Build history of the part. All positions in model axes, mm. A direction names the side the tool comes from. Round coordinates to 2 decimals unless told otherwise and drop trailing zeros. Order: outer loops, then holes, each group sorted by start corner. A loop starts at its lowest first (then second) coordinate and runs counter-clockwise, first axis right, second up. Notation, with made-up numbers: (38, -14.5) -> (83, -14.5) arc R21 cw to (83, 21.5) -> close; hole circle Ø4 at (89.5, -0.75). An arc over 180 degrees is marked (long way). Answer as a JSON object with one key per item and string values.
from build123d import *

# Parameters (mm, degrees)
SKETCH1_W           = 42
SKETCH1_H           = 42
BOSS_EXTRUDE1_DEPTH = 6
SKETCH2_W           = 39
SKETCH2_H           = 39
CUT_EXTRUDE1_DEPTH  = 3.5
CUT_EXTRUDE2_REACH  = 31.904
SKETCH3_W           = 5
SKETCH3_H           = 7
SKETCH3_W_2         = 13
SKETCH3_H_2         = 6
BOSS_EXTRUDE2_DEPTH = 2
SKETCH5_R           = 1
CUT_EXTRUDE3_DEPTH  = 31.037476592
SKETCH6_R           = 5
BOSS_EXTRUDE3_DEPTH = 8
SKETCH7_R           = 2.5
BOSS_EXTRUDE4_DEPTH = 10
FILLET1_R           = 1


with BuildPart() as part:
    # Sketch1 → Boss-Extrude1 (new body)
    with BuildSketch(Plane(origin=(0, 0, 0), x_dir=(1, 0, 0), z_dir=(0, 1, 0))):
        Rectangle(SKETCH1_W, SKETCH1_H)
    extrude(amount=BOSS_EXTRUDE1_DEPTH)

    # Sketch2 → Cut-Extrude1 (cut)
    with BuildSketch(Plane.XZ):
        Rectangle(SKETCH2_W, SKETCH2_H)
    extrude(amount=-CUT_EXTRUDE1_DEPTH, mode=Mode.SUBTRACT)

    # Sketch3 → Cut-Extrude2 (cut, up to next)
    with BuildSketch(Plane.XZ.offset(-3.5), mode=Mode.PRIVATE) as cut_extrude2_sk1:
        with Locations((-17, 8.5)):
            Rectangle(SKETCH3_W, SKETCH3_H)
    cut_extrude2_tool1 = extrude(cut_extrude2_sk1.sketch, amount=-CUT_EXTRUDE2_REACH, mode=Mode.PRIVATE) & part.part
    # Sketch3 → Cut-Extrude2 (cut, up to next)
    with BuildSketch(Plane.XZ.offset(-3.5), mode=Mode.PRIVATE) as cut_extrude2_sk2:
        with Locations((-6, 16.5)):
            Rectangle(SKETCH3_W_2, SKETCH3_H_2)
    cut_extrude2_tool2 = extrude(cut_extrude2_sk2.sketch, amount=-CUT_EXTRUDE2_REACH, mode=Mode.PRIVATE) & part.part
    add(cut_extrude2_tool1.solids().sort_by_distance((-17, 3.5, 8.5))[0], mode=Mode.SUBTRACT)
    add(cut_extrude2_tool2.solids().sort_by_distance((-6, 3.5, 16.5))[0], mode=Mode.SUBTRACT)

    # Sketch4 → Boss-Extrude2 (add)
    with BuildSketch(Plane.XZ.offset(-3.5)):
        with BuildLine():
            Line((-19.5, 17), (-19.5, 19.5))
            Line((-19.5, 19.5), (-17, 19.5))
            ThreePointArc((-17, 19.5), (-15.232233047, 15.232233047), (-19.5, 17))
        make_face()
        with BuildLine():
            Line((19.5, 19.5), (17, 19.5))
            ThreePointArc((17, 19.5), (15.232233047, 15.232233047), (19.5, 17))
            Line((19.5, 17), (19.5, 19.5))
        make_face()
        with BuildLine():
            Line((-19.5, -19.5), (-17, -19.5))
            ThreePointArc((-17, -19.5), (-15.232233047, -15.232233047), (-19.5, -17))
            Line((-19.5, -17), (-19.5, -19.5))
        make_face()
        with BuildLine():
            Line((19.5, -17), (19.5, -19.5))
            Line((19.5, -19.5), (17, -19.5))
            ThreePointArc((17, -19.5), (15.232233047, -15.232233047), (19.5, -17))
        make_face()
    extrude(amount=BOSS_EXTRUDE2_DEPTH)

    # Sketch5 → Cut-Extrude3 (cut, through all)
    with BuildSketch(Plane.XZ.offset(-1.5)):
        with Locations(Location((-17, 17, 0), (0, 0, 270))):
            Circle(SKETCH5_R)
        with Locations(Location((17, 17, 0), (0, 0, 270))):
            Circle(SKETCH5_R)
        with Locations(Location((17, -17, 0), (0, 0, 270))):
            Circle(SKETCH5_R)
        with Locations(Location((-17, -17, 0), (0, 0, 270))):
            Circle(SKETCH5_R)
    extrude(amount=-CUT_EXTRUDE3_DEPTH, mode=Mode.SUBTRACT)

    # Sketch6 → Boss-Extrude3 (add)
    with BuildSketch(Plane(origin=(0, 6, 0), x_dir=(1, 0, 0), z_dir=(0, 1, 0))):
        with Locations(Location((0, 0, 0), (0, 0, 270))):
            Circle(SKETCH6_R)
    extrude(amount=BOSS_EXTRUDE3_DEPTH)

    # Sketch7 → Boss-Extrude4 (add)
    with BuildSketch(Plane(origin=(0, 14, 0), x_dir=(1, 0, 0), z_dir=(0, 1, 0))):
        with Locations(Location((0, 0, 0), (0, 0, 270))):
            Circle(SKETCH7_R)
    extrude(amount=BOSS_EXTRUDE4_DEPTH)

    # Fillet1
    fillet1_edges = [part.edges().sort_by_distance(p)[0] for p in [
        (0, 6, -5),
        (0, 14, -2.5),
        (0, 24, -2.5),
        (-21, 6, 0),
        (0, 6, 21),
        (-14.5, 4.75, 12),
        (-14.5, 4.75, 5),
        (-19.5, 4.75, 5),
        (-19.5, 4.75, 12),
        (0.5, 4.75, 19.5),
        (0.5, 4.75, 13.5),
        (-12.5, 4.75, 13.5),
        (-12.5, 4.75, 19.5),
        (21, 6, 0),
        (21, 3, 21),
        (-21, 3, 21),
        (-21, 3, -21),
        (21, 3, -21),
        (0, 6, -21),
    ]]
    fillet(fillet1_edges, radius=FILLET1_R)


solid = part.part
1) Probe L1, parallel to X at y = 3.9, z = 17; L2, parallel to X at y = 4.7, z = -17; L3, parallel to X at y = 3, z = 4.5. List the from-to ranges inside material, lowest first. Write a range as from..to.
Checked values:
{"L1": "x = -21..-18, -16..-12.5, 0.5..16, 18..21", "L2": "x = -21..-18, -16..16, 18..21", "L3": "x = -21..-19.5, 19.5..21"}
2) Which spindle directions (+Z, -Z, +X, -X, +Y, -Y) get a long thin tool onto all of the face, cutting with end or side? Do faces 5 (the face through (0, 2, 21)), 6 (the face through (-14.801, 4.768, 11.715)), 7 (the face through (-18, 1.5, 18)). Say none if no direction does.
Checked values:
{"face 5": "+Z, +X, -X, +Y, -Y", "face 6": "+Y, -Y", "face 7": "-Y"}
3) Pull direction Z, two halves, no side cores. Call faces 1 (the face through (20.699, 2.535, 20.715)), 2 (the face through (0.215, 4.768, 13.801)), 3 (the face through (0, 2, -19.5)), 4 (the face through (-20.699, 5.715, -0.28)): pulls with the +Z half, pulls with the -Z half, needs draft (parallel to the pull), parting line crosses it, or undercut.
Checked values:
{"face 1": "pulls with the +Z half", "face 2": "undercut", "face 3": "undercut", "face 4": "needs draft"}
4) Cut at A-A, the plane y = 2.5. Give the cut face in (x, z), plus the area to 3 significant figures.
Checked values:
{"outline": "(-21, -20) arc R1 ccw to (-20, -21) -> (20, -21) arc R1 ccw to (21, -20) -> (21, 20) arc R1 ccw to (20, 21) -> (-20, 21) arc R1 ccw to (-21, 20) -> close; hole (-19.5, -17) arc R2.5 cw (long way) to (-17, -19.5) -> (17, -19.5) arc R2.5 cw (long way) to (19.5, -17) -> (19.5, 17) arc R2.5 cw (long way) to (17, 19.5) -> (-17, 19.5) arc R2.5 cw (long way) to (-19.5, 17) -> close; hole circle Ø2 at (-17, -17); hole circle Ø2 at (-17, 17); hole circle Ø2 at (17, -17); hole circle Ø2 at (17, 17)", "area": "313 mm²"}
5) Cut at B-B, the plane z = 7. Give the cut face in (x, y).
Checked values:
{"outline": "(-21, 0) -> (-19.5, 0) -> (-19.5, 6) -> (-20, 6) arc R1 ccw to (-21, 5) -> close; (-14.5, 3.5) -> (19.5, 3.5) -> (19.5, 0) -> (21, 0) -> (21, 5) arc R1 ccw to (20, 6) -> (-14.5, 6) -> close"}
6) Cut at D-D, the plane z = -9.5. Give the cut face in (x, y).
Checked values:
{"outline": "(-21, 0) -> (-19.5, 0) -> (-19.5, 3.5) -> (19.5, 3.5) -> (19.5, 0) -> (21, 0) -> (21, 5) arc R1 ccw to (20, 6) -> (-20, 6) arc R1 ccw to (-21, 5) -> close"}
7) Flat gauge pins, fed straight in: pin 1 Ø2 at (y, z) = (5.5, 7.5) entering from -X; pin 2 Ø12 at (x, y) = (4, 12.5) entering from -Z; pin 3 Ø2 at (x, z) = (-6, -10) entering from +Y; pin 4 Ø1.5 at (x, z) = (-16.5, -17) entering from -Y. Where does each tip first touch, or does it go through?
Checked values:
{"pin 1": "stops at x = -21", "pin 2": "stops at z = -5", "pin 3": "stops at y = 6", "pin 4": "stops at y = 1.5"}
8) Cut at C-C, the plane x = 8.5. Give the cut face in (y, z).
Checked values:
{"outline": "(0, -21) -> (5, -21) arc R1 ccw to (6, -20) -> (6, 20) arc R1 ccw to (5, 21) -> (0, 21) -> (0, 19.5) -> (3.5, 19.5) -> (3.5, -19.5) -> (0, -19.5) -> close"}
